Autodesk Inventor part; units mm, degrees
ref_plane "YZ Plane" through (0, 0, 0) normal (1, 0, 0) x (0, 1, 0)
ref_plane "XZ Plane" through (0, 0, 0) normal (0, 1, 0) x (-1, 0, 0)
ref_plane "XY Plane" through (0, 0, 0) normal (0, 0, 1) x (1, 0, 0)
sketch "Эскиз1" plane through (0, 0, 0) normal (0, 1, 0) x (-1, 0, 0)
  line L0 (0, 0) -> (0, -10)
  line L1 (0, -10) -> (-5, -10)
  line L2 (-5, -10) -> (-5, -20)
  line L3 (-5, -20) -> (-5, 0)
  line L4 (-5, 0) -> (0, 0)
  line L5 (-5, 0) -> (-5, 10)
  line L6 (-5, 0) -> (-15, 0)
  line L7 (-15, 0) -> (-5, 10)
  line L8 (-15, 0) -> (-15, -10)
  line L9 (-15, -10) -> (-5, -20)
  dimension "d2" = 10
  dimension "d3" = 5
  dimension "d4" = 10
  dimension "d5" = 10
  dimension "d6" = 10
extrude "Выдавливание1" add sketch "Эскиз1" along normal blind 60
properties part number "Dyenhtyytt cjtlbytybt"
CAD build for the part. Positions are in the model's coordinates, mm. A direction names the side the tool comes from. Round coordinates to 2 decimals unless told otherwise and drop trailing zeros. Order: outer loops, then holes, each group sorted by start corner. A loop starts at its lowest first (then second) coordinate and runs counter-clockwise, first axis right, second up. Notation, with made-up numbers: (18.5, 71.5) -> (36.5, 71.5) arc R26 cw to (36.5, 95.5) -> close; hole circle Ø2 at (50.5, 61). An arc over 180 degrees is marked (long way). Write each question's results on one line, items separated by ' | '.
1. Wall check: line 1 along Z through (x, y) = (1.5, 41.5); line 2 along X through (y, z) = (21, -12); line 3 along X through (y, z) = (57, 3). Give the ranges that are in metal, low to high. Write a range as [from, to].
Findings below:
line 1: z = [-10, 0] | line 2: x = [5, 13] | line 3: x = [5, 12]
2. Cut at B-B (x = 11.25). Give the cut face in (y, z).
Findings below:
outline: (0, -13.75) -> (60, -13.75) -> (60, 3.75) -> (0, 3.75) -> close
3. Cut at C-C (z = 8). Give the cut face in (x, y).
Findings below:
outline: (5, 0) -> (7, 0) -> (7, 60) -> (5, 60) -> close
4. Cut at A-A (y = 40). Give the cut face in (x, z).
Findings below:
outline: (0, -10) -> (5, -10) -> (5, -20) -> (15, -10) -> (15, 0) -> (5, 10) -> (5, 0) -> (0, 0) -> close
5. Flat gauge pins, fed straight in: P1, Ø8, axis at y = 27.5, z = 5.5, coming from the -X side; P2, Ø5.5, axis at x = 1.5, y = 27.5, coming from the +Z side; P3, Ø6, axis at y = 42, z = -10.5, coming from the -X side; P4, Ø1.5, axis at x = 2, y = 23, coming from the -Z side. Where does each tip first touch, or does it go through?
Findings below:
P1: stops at x = 5 | P2: stops at z = 0 | P3: stops at x = 0 | P4: stops at z = -10
6. 3-axis set-ups, long thin cutter, end or side, ignore diameter. For faces 1 (the face through (10, 30, -15)), 2 (the face through (5, 30, -15)), 3 (the face through (5, 30, 5)): which of +Z, -Z, +X, -X, +Y, -Y reach the whole face in a straight line?
Findings below:
face 1: -Z, +X, +Y, -Y | face 2: -Z, -X, +Y, -Y | face 3: +Z, -X, +Y, -Y
